from build123d import *
from build123d.topology import SkipClean

# Parameters (mm, degrees)
SKETCH1_W           = 28
SKETCH1_H           = 31
BOSS_EXTRUDE1_DEPTH = 7.425
SKETCH2_R           = 1.25
BOSS_EXTRUDE2_DEPTH = 0.5
BOSS_EXTRUDE3_DEPTH = 1.525
SKETCH3_R           = 12.7
CUT_EXTRUDE1_DEPTH  = 0.635
SKETCH7_R           = 0.6
BOSS_EXTRUDE6_DEPTH = 2.5


with BuildPart() as part:
    # Sketch1 → Boss-Extrude1 (new, symmetric)
    with BuildSketch(Plane(origin=(0, 0, 0), x_dir=(1, 0, 0), z_dir=(0, 1, 0))):
        with Locations((14, 15.5)):
            Rectangle(SKETCH1_W, SKETCH1_H)
    extrude(amount=BOSS_EXTRUDE1_DEPTH, both=True)

    # Sketch2 → Boss-Extrude2 (add, symmetric)
    # profile 1 of 2: a face of its own
    with BuildSketch(Plane(origin=(0, 0, 0), x_dir=(1, 0, 0), z_dir=(0, 1, 0))):
        with BuildLine():
            Line((0, 8.7), (0, 22.3))
            Line((0, 22.3), (-6.386291535, 18.509844274))
            ThreePointArc((-6.386291535, 18.509844274), (-8.1, 15.5), (-6.386291535, 12.490155726))
            Line((-6.386291535, 12.490155726), (0, 8.7))
        make_face()
        with Locations(Location((-4.6, 15.5, 0), (0, 0, 270))):
            Circle(SKETCH2_R, mode=Mode.SUBTRACT)
    # profile 2 of 2: a face of its own
    with BuildSketch(Plane(origin=(0, 0, 0), x_dir=(1, 0, 0), z_dir=(0, 1, 0))):
        with BuildLine():
            Line((34.386291535, 12.490155726), (28, 8.7))
            Line((28, 8.7), (28, 22.3))
            Line((28, 22.3), (34.386291535, 18.509844274))
            ThreePointArc((34.386291535, 18.509844274), (36.1, 15.5), (34.386291535, 12.490155726))
        make_face()
        with Locations(Location((32.6, 15.5, 0), (0, 0, 90))):
            Circle(SKETCH2_R, mode=Mode.SUBTRACT)
    extrude(amount=BOSS_EXTRUDE2_DEPTH, both=True)

    # Sketch5 → Boss-Extrude3 (add, symmetric)
    with SkipClean():  # the faces are left unmerged after this step: merging them gives an invalid solid
        with BuildSketch(Plane(origin=(0, 0, 0), x_dir=(1, 0, 0), z_dir=(0, 1, 0))):
            with BuildLine():
                ThreePointArc((-6.386291535, 18.509844274), (-8.1, 15.5), (-6.386291535, 12.490155726))
                Line((-6.386291535, 12.490155726), (0, 8.7))
                Line((0, 8.7), (0, 9.659933384))
                Line((0, 9.659933384), (-0.8255, 10.149853635))
                Line((-0.8255, 10.149853635), (-5.964981917, 13.200048997))
                ThreePointArc((-5.964981917, 13.200048997), (-7.2745, 15.5), (-5.964981917, 17.799951003))
                Line((-5.964981917, 17.799951003), (-0.8255, 20.850146365))
                Line((-0.8255, 20.850146365), (0, 21.340066616))
                Line((0, 21.340066616), (0, 22.3))
                Line((0, 22.3), (-6.386291535, 18.509844274))
            make_face()
            with BuildLine():
                ThreePointArc((34.386291535, 12.490155726), (36.1, 15.5), (34.386291535, 18.509844274))
                Line((34.386291535, 18.509844274), (28, 22.3))
                Line((28, 22.3), (28, 21.340066616))
                Line((28, 21.340066616), (28.8255, 20.850146365))
                Line((28.8255, 20.850146365), (33.964981917, 17.799951003))
                ThreePointArc((33.964981917, 17.799951003), (35.2745, 15.5), (33.964981917, 13.200048997))
                Line((33.964981917, 13.200048997), (28.8255, 10.149853635))
                Line((28.8255, 10.149853635), (28, 9.659933384))
                Line((28, 9.659933384), (28, 8.7))
                Line((28, 8.7), (34.386291535, 12.490155726))
            make_face()
        extrude(amount=BOSS_EXTRUDE3_DEPTH, both=True)
    add(part.part.scale(1), mode=Mode.REPLACE)  # the faces are merged on a copy

    # Sketch3 → Cut-Extrude1 (cut)
    with BuildSketch(Plane(origin=(0, 7.425, 0), x_dir=(1, 0, 0), z_dir=(0, 1, 0))):
        with Locations(Location((14, 15.5, 0), (0, 0, 270))):
            Circle(SKETCH3_R)
    extrude(amount=-CUT_EXTRUDE1_DEPTH, mode=Mode.SUBTRACT)

    # Sketch6 → Revolve1 (revolve)
    with BuildSketch(Plane(origin=(0, 0, -15.5), x_dir=(-1, 0, 0), z_dir=(0, 0, -1)), mode=Mode.PRIVATE) as revolve1_sk:
        with BuildLine():
            Line((-22.493511176, 6.79), (-22.810948315, 7.046589007))
            ThreePointArc((-22.810948315, 7.046589007), (-22.816802833, 7.372772527), (-22.494598431, 7.321642421))
            ThreePointArc((-22.494598431, 7.321642421), (-22.403694623, 7.232370162), (-22.280839201, 7.198612444))
            ThreePointArc((-22.280839201, 7.198612444), (-18.140521992, 7.154934635), (-14, 7.140375125))
            Line((-14, 7.140375125), (-14, 6.79))
            Line((-14, 6.79), (-22.493511176, 6.79))
        make_face()
        with BuildLine():
            Line((-26.083336466, 6.79), (-22.86, 6.79))
            ThreePointArc((-22.86, 6.79), (-24.471668233, 7.315802401), (-26.083336466, 6.79))
        make_face()
    revolve(revolve1_sk.sketch.rotate(Axis((14, -7.425, -15.5), (0, 1, 0)), 90), axis=Axis((14, -7.425, -15.5), (0, 1, 0)))

    # Sketch7 → Boss-Extrude6 (add)
    with BuildSketch(Plane.XY):
        with Locations(Location((14.625, 3.925, 0), (0, 0, 180))):
            Circle(SKETCH7_R)
        with Locations(Location((13.375, 3.925, 0), (0, 0, 180))):
            Circle(SKETCH7_R)
    extrude(amount=BOSS_EXTRUDE6_DEPTH)


solid = part.part
Source: CAD feature listing. Evaluate the final solid. Frame: model axes, mm. A direction names the side the tool comes from. Give positions to 0.01 mm unless a question says otherwise; leave off trailing zeros. Write each loop counter-clockwise with the first axis right and the second up, starting at its lowest first coordinate (ties: lowest second). Pieces come first, ordered by that corner, then holes. Notation, with made-up numbers: M 3,-35.5 L 38,-35.5 A11 cw 38,-23.5 Z; hole C -39.75,-22.5 d3. An arc over 180 degrees is marked long. Return JSON: item names as keys, results as strings. Group by question number.
1) Cut plane B-B, the plane y = 2.5. Output: boundary loops of the cut face in (x, z).
2) Material intervals for line 1 along Y through (x, z) = (11, -4.5) (3 decimals); line 2 along Y through (x, z) = (15, -26) (3 decimals); line 3 along X through (y, z) = (-3, -11.5), sorted ascending. Write a range as [from, to].
3) Set-up query: faces 4 (the face through (-6, 1.525, -13)), 5 (the face through (-3.2, 0, -10.6)), 6 (the face through (-6, -1.525, -13)), 7 (the face through (-3, 0.5, -16)). Return all of +Z, -Z, +X, -X, +Y, -Y with unobstructed straight access to the full face (end or side cutting, diameter ignored); none if empty.
4) Cut plane A-A, the plane x = -4.6. Output: boundary loops of the cut face in (y, z) (3 decimals).
5) Pull-direction query (Z, two-part tool) for faces 1 (the face through (14.3, 3.42, 1.23)), 2 (the face through (31.2, 0, -20.4)), 3 (the face through (9, 6.79, -4)); classes: pulls with the +Z half, pulls with the -Z half, needs draft (parallel to the pull), parting line crosses it, or undercut.
6) Pin query (flat end, axial travel): P1, Ø1.5, axis at x = 31, y = -1.5, coming from the +Z side; P2, Ø3, axis at x = 23.5, z = -12, coming from the +Y side (3 decimals); P3, Ø2, axis at x = 33.5, z = -15, coming from the +Y side; P4, Ø2, axis at x = 30, y = 0, coming from the +Z side. Return the tip coordinate at first contact, or that it passes through.
7) Cut plane C-C, the plane z = -15.5. Give the number of separate pieces and of enclosed holes in the cut face, plus the area to 3 significant figures.
Recorded:
{
 "1": {"outline": "M 0,-31 L 28,-31 L 28,0 L 0,0 Z"},
 "2": {"line 1": "y = [-7.425, 7.153]", "line 2": "y = [-7.425, 7.315]", "line 3": "x = [0, 28]"},
 "3": {"face 4": "+Z, -Z, -X, +Y", "face 5": "+Z, -X, +Y, -Y", "face 6": "+Z, -Z, -X, -Y", "face 7": "+Y"},
 "4": {"outline": "M -1.525,-19.57 L 1.525,-19.57 L 1.525,-18.61 L 0.5,-18.61 L 0.5,-16.75 L -0.5,-16.75 L -0.5,-18.61 L -1.525,-18.61 Z; M -1.525,-12.39 L -0.5,-12.39 L -0.5,-14.25 L 0.5,-14.25 L 0.5,-12.39 L 1.525,-12.39 L 1.525,-11.43 L -1.525,-11.43 Z"},
 "5": {"face 1": "needs draft", "face 2": "pulls with the -Z half", "face 3": "undercut"},
 "6": {"P1": "stops at z = -10.04", "P2": "stops at y = 7.425", "P3": "stops at y = 0.5", "P4": "stops at z = -9.29"},
 "7": {"separate pieces": "3", "enclosed holes": "0", "area": "423 mm²"}
}
